Check sheet for the drawn part. Datum: minimum x, y, z corner. Units: mm. Round coordinates to 2 decimals unless told otherwise and drop trailing zeros. Write each loop counter-clockwise with the first axis right and the second up, starting at its lowest first coordinate (ties: lowest second). Pieces come first, ordered by that corner, then holes. Notation, with made-up numbers: M 57,67.5 L 67,67.5 A22 cw 67,88.5 Z; hole C 79.25,29 d11. An arc over 180 degrees is marked long. One line per item, written item: value. Start each with the question number.
Item 1: Section check A-A, the plane z = 2.5. State how many separate pieces and enclosed holes the cut face has, then the cut area to 3 significant figures.
Item 2: Section check B-B, the plane x = 75. Record the cut outline in (y, z).
Item 3: Thickness scan on probe 1 along Y at (x, z) = (10.5, 5.5) (1 decimal); probe 2 along Y at (x, z) = (34.5, 4); probe 3 along X at (y, z) = (23.5, 0.5). Record the ranges inside material, lowest first. Write a range as from..to.
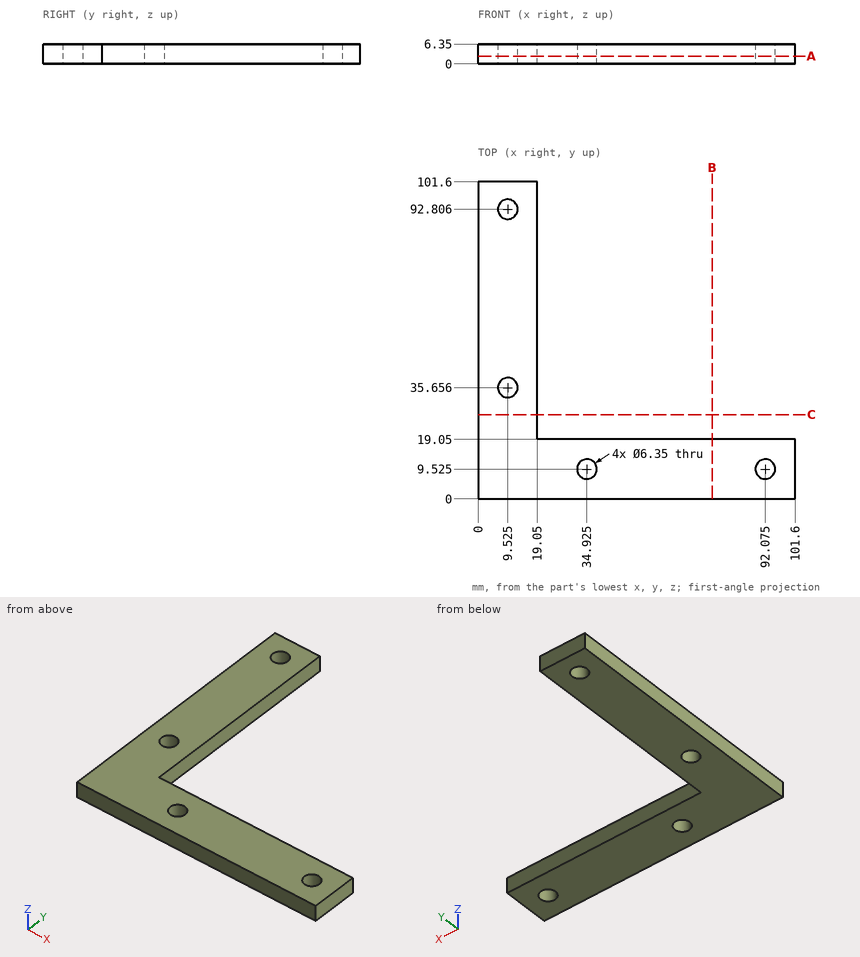
Response values:
1. separate pieces: 1
1. enclosed holes: 4
1. area: 3,380 mm2
2. outline: M 0,0 L 19.05,0 L 19.05,6.35 L 0,6.35 Z
3. probe 1: y = 0..32.6, 38.7..89.8, 95.8..101.6
3. probe 2: y = 0..6.38, 12.67..19.05
3. probe 3: x = 0..19.05
